The listing builds one solid part. Answer for the finished solid, in the listing's coordinates (mm). Give positions to 0.01 mm unless a question says otherwise; leave off trailing zeros. Order: outer loops, then holes, each group sorted by start corner. A loop starts at its lowest first (then second) coordinate and runs counter-clockwise, first axis right, second up. Notation, with made-up numbers: (31, 80.25) -> (86, 80.25) arc R36 ccw to (86, 116.25) -> close; hole circle Ø11 at (-24.75, 86.25). An arc over 180 degrees is marked (long way). Write item = value, one per line. Start each with the question number.
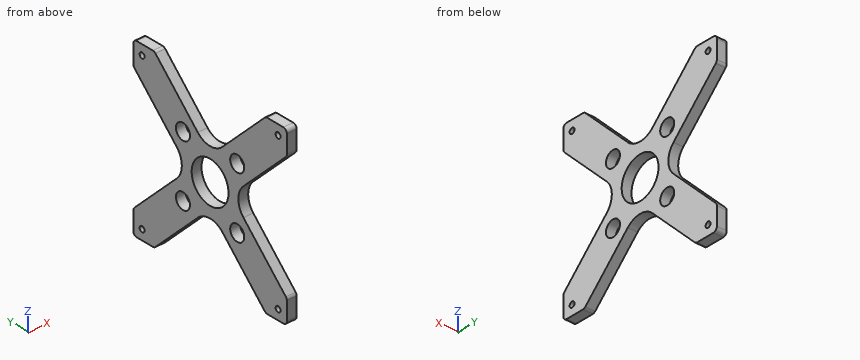
```python
from build123d import *

# Parameters (mm, degrees)
BOSS_EXTRUDE1_DEPTH     = 6.35
SKETCH1_9_R             = 13.335
CUT_EXTRUDE1_DEPTH      = 11.938
SKETCH1_10_R            = 1.778
CUT_EXTRUDE2_DEPTH      = 24.638
SKETCH1_11_R            = 1.778
CUT_EXTRUDE3_DEPTH      = 24.13
SKETCH1_12_R            = 1.778
CUT_EXTRUDE4_DEPTH      = 38.862
SKETCH1_13_R            = 1.778
CUT_EXTRUDE5_DEPTH      = 13.462
FILLET1_R               = 2.54
SKETCH2_R               = 5.08
CUT_EXTRUDE6_DEPTH      = 13.462
MIRROR2_COPY_1_SKETCH_R = 5.08
MIRROR2_COPY_1_DEPTH    = 13.462


with BuildPart() as part:
    # Sketch1 → Boss-Extrude1 (new body)
    with BuildSketch(Plane(origin=(0, 0, 0), x_dir=(0, 0, -1), z_dir=(1, 0, 0))):
        with BuildLine():
            Line((-53.874845122, 46.825199553), (-38.634845122, 46.825199553))
            Line((-38.634845122, 46.825199553), (-7.203948698, 15.394303129))
            ThreePointArc((-7.203948698, 15.394303129), (1.709004986, 11.702436832), (10.621958671, 15.394303129))
            Line((10.621958671, 15.394303129), (42.052855095, 46.825199553))
            Line((42.052855095, 46.825199553), (57.292855095, 46.825199553))
            Line((57.292855095, 46.825199553), (57.292855095, 31.585199553))
            Line((57.292855095, 31.585199553), (25.861958671, 0.154303129))
            ThreePointArc((25.861958671, 0.154303129), (22.170092374, -8.758650555), (25.861958671, -17.67160424))
            Line((25.861958671, -17.67160424), (57.292855095, -49.102500664))
            Line((57.292855095, -49.102500664), (57.292855095, -64.342500664))
            Line((57.292855095, -64.342500664), (42.052855095, -64.342500664))
            Line((42.052855095, -64.342500664), (10.621958671, -32.91160424))
            ThreePointArc((10.621958671, -32.91160424), (1.709004986, -29.219737943), (-7.203948698, -32.91160424))
            Line((-7.203948698, -32.91160424), (-38.634845122, -64.342500664))
            Line((-38.634845122, -64.342500664), (-53.874845122, -64.342500664))
            Line((-53.874845122, -64.342500664), (-53.874845122, -49.102500664))
            Line((-53.874845122, -49.102500664), (-22.443948698, -17.67160424))
            ThreePointArc((-22.443948698, -17.67160424), (-18.752082401, -8.758650555), (-22.443948698, 0.154303129))
            Line((-22.443948698, 0.154303129), (-53.874845122, 31.585199553))
            Line((-53.874845122, 31.585199553), (-53.874845122, 46.825199553))
        make_face()
    extrude(amount=BOSS_EXTRUDE1_DEPTH)

    # Sketch1<9> → Cut-Extrude1 (cut)
    with BuildSketch(Plane(origin=(0, 0, 0), x_dir=(0, 0, -1), z_dir=(1, 0, 0))):
        with Locations((1.709004986, -8.758650555)):
            Circle(SKETCH1_9_R)
    extrude(amount=CUT_EXTRUDE1_DEPTH, mode=Mode.SUBTRACT)

    # Sketch1<10> → Cut-Extrude2 (cut)
    with BuildSketch(Plane(origin=(0, 0, 0), x_dir=(0, 0, -1), z_dir=(1, 0, 0))):
        with Locations((-47.503495014, -57.971150555)):
            Circle(SKETCH1_10_R)
    extrude(amount=CUT_EXTRUDE2_DEPTH, mode=Mode.SUBTRACT)

    # Sketch1<11> → Cut-Extrude3 (cut)
    with BuildSketch(Plane(origin=(0, 0, 0), x_dir=(0, 0, -1), z_dir=(1, 0, 0))):
        with Locations((50.921504986, -57.971150555)):
            Circle(SKETCH1_11_R)
    extrude(amount=CUT_EXTRUDE3_DEPTH, mode=Mode.SUBTRACT)

    # Sketch1<12> → Cut-Extrude4 (cut)
    with BuildSketch(Plane(origin=(0, 0, 0), x_dir=(0, 0, -1), z_dir=(1, 0, 0))):
        with Locations((50.921504986, 40.453849445)):
            Circle(SKETCH1_12_R)
    extrude(amount=CUT_EXTRUDE4_DEPTH, mode=Mode.SUBTRACT)

    # Sketch1<13> → Cut-Extrude5 (cut)
    with BuildSketch(Plane(origin=(0, 0, 0), x_dir=(0, 0, -1), z_dir=(1, 0, 0))):
        with Locations((-47.503495014, 40.453849445)):
            Circle(SKETCH1_13_R)
    extrude(amount=CUT_EXTRUDE5_DEPTH, mode=Mode.SUBTRACT)

    # Fillet1
    fillet1_edges = [part.edges().sort_by_distance(p)[0] for p in [
        (3.175, 46.825199553, 53.874845122),
        (3.175, 46.825199553, 38.634845122),
        (3.175, 46.825199553, -42.052855095),
        (3.175, 46.825199553, -57.292855095),
        (3.175, 31.585199553, -57.292855095),
        (3.175, -49.102500664, -57.292855095),
        (3.175, -64.342500664, -57.292855095),
        (3.175, -64.342500664, -42.052855095),
        (3.175, -64.342500664, 38.634845122),
        (3.175, -64.342500664, 53.874845122),
        (3.175, -49.102500664, 53.874845122),
        (3.175, 31.585199553, 53.874845122),
    ]]
    fillet(fillet1_edges, radius=FILLET1_R)

    # Sketch2 → Cut-Extrude6 (cut)
    with BuildSketch(Plane.ZY):
        with Locations((-21.351416825, 10.883761284)):
            Circle(SKETCH2_R)
    cut_extrude6 = extrude(amount=-CUT_EXTRUDE6_DEPTH, mode=Mode.SUBTRACT)

    # Mirror1: Cut-Extrude6 across plane
    add(cut_extrude6.mirror(Plane.ZX.offset(-8.758650555)), mode=Mode.SUBTRACT)

    # Mirror2: Cut-Extrude6 across plane
    add(cut_extrude6.mirror(Plane.XY.offset(-1.709004986)), mode=Mode.SUBTRACT)

    # Mirror2 copy 1 sketch → Mirror2 copy 1 (cut)
    with BuildSketch(Plane(origin=(0, -17.517301111, -3.418009973), x_dir=(0, 0, -1), z_dir=(-1, 0, 0))):
        with Locations((-21.351416825, 10.883761284)):
            Circle(MIRROR2_COPY_1_SKETCH_R)
    extrude(amount=-MIRROR2_COPY_1_DEPTH, mode=Mode.SUBTRACT)


solid = part.part
```
Item 1: Consider L1, parallel to Z at x = 2.75, y = -59.5; L2, parallel to Z at x = 1, y = 39; L3, parallel to Z at x = 1.5, y = -53. Determine where each line is inside the solid, lowest interval first. Write a range as from..to.
Item 2: Flat-ended cylindrical pins translate along their axes: pin 1 (1.5 mm diameter, centred on x = 3, y = -44, fed in from -Z); pin 2 (1 mm diameter, centred on x = 4, z = 32, fed in from +Y); pin 3 (2 mm diameter, centred on x = 5, y = -24.5, fed in from +Z). Find the tip coordinate at first contact, or state that the pin passes through.
Item 3: A cutting plane is placed at C-C, the plane z = -20.5. Write down the section's boundary in (x, y), plus the area to 3 significant figures.
Item 4: A cutting plane is placed at A-A, the plane y = -35.5. Write down the section's boundary in (x, z), plus the area to 3 significant figures.
Item 5: A cutting plane is placed at D-D, the plane x = 1.5. Count the separate pieces of the cut face and the enclosed holes in it, plus the area to 3 significant figures.
Item 6: A cutting plane is placed at B-B, the plane z = 30. Write down the section's boundary in (x, y), plus the area to 3 significant figures.
Check values:
q1.L1 = -57.29..-51.83, -50.01..-37.21, 33.79..46.6, 48.41..53.87
q1.L2 = -57.29..-51.95, -49.9..-34.23, 30.81..46.48, 48.53..53.87
q1.L3 = -57.29..-30.71, 27.29..53.87
q2.pin_1 = -52.94
q2.pin_2 = 40.69
q2.pin_3 = 30.27
q3.outline = (0, -42.79) -> (6.35, -42.79) -> (6.35, -33.41) -> (0, -33.41) -> close; (0, -23.39) -> (6.35, -23.39) -> (6.35, 5.88) -> (0, 5.88) -> close; (0, 15.89) -> (6.35, 15.89) -> (6.35, 25.27) -> (0, 25.27) -> close
q3.area = 305 mm^2
q4.outline = (0, -43.69) -> (6.35, -43.69) -> (6.35, -13.21) -> (0, -13.21) -> close; (0, 9.79) -> (6.35, 9.79) -> (6.35, 40.27) -> (0, 40.27) -> close
q4.area = 387 mm^2
q5.separate_pieces = 1
q5.enclosed_holes = 9
q5.area = 5,050 mm^2
q6.outline = (0, -55.71) -> (6.35, -55.71) -> (6.35, -25.23) -> (0, -25.23) -> close; (0, 7.71) -> (6.35, 7.71) -> (6.35, 38.19) -> (0, 38.19) -> close
q6.area = 387 mm^2
